```python
from build123d import *

# Parameters (mm, degrees)
SKETCH2_W                    = 28
SKETCH2_H                    = 8
BOSS_EXTRUDE1_DEPTH          = 2
SKETCH3_R                    = 2.35
BOSS_EXTRUDE2_DEPTH          = 10
CHAMFER1_SIZE                = 10
CHAMFER1_SIZE_2              = 0.3
LPATTERN1_COUNT              = 2
LPATTERN1_PITCH              = 20
CHAMFER1_OF_LPATTERN1_SIZE   = 10
CHAMFER1_OF_LPATTERN1_SIZE_2 = 0.3


with BuildPart() as part:
    # Sketch2 → Boss-Extrude1 (new body)
    with BuildSketch(Plane(origin=(0, 0, 0), x_dir=(1, 0, 0), z_dir=(0, 1, 0))):
        Rectangle(SKETCH2_W, SKETCH2_H)
    extrude(amount=BOSS_EXTRUDE1_DEPTH)

    # Sketch3 → Boss-Extrude2 (add)
    with BuildSketch(Plane(origin=(0, 2, 0), x_dir=(1, 0, 0), z_dir=(0, 1, 0))):
        with Locations(Location((10, 0, 0), (0, 0, 90))):
            Circle(SKETCH3_R)
    boss_extrude2 = extrude(amount=BOSS_EXTRUDE2_DEPTH)

    # Chamfer1
    # the kernel refuses this chamfer: 10, 0.3 mm, written as the material it takes off along each edge
    with BuildSketch(Plane(origin=(10, 12, 0), x_dir=(0, 0, -1), z_dir=(1, 0, 0))) as chamfer1_piece_1_section:
        Polygon((2.35, -CHAMFER1_SIZE), (2.35 - CHAMFER1_SIZE_2, 0), (2.35, 0), align=None)
    chamfer1_piece_1 = revolve(axis=Axis((10, 12, 0), (0, 1, 0)), mode=Mode.PRIVATE)
    chamfer1_piece_1 = split(chamfer1_piece_1, bisect_by=Plane(origin=(10, 2, 2.231636086), z_dir=(0, 1, 0)), keep=Keep.TOP, mode=Mode.PRIVATE)
    add(chamfer1_piece_1, mode=Mode.SUBTRACT)

    # LPattern1: Boss-Extrude2 ×2
    with Locations(*[(-i * LPATTERN1_PITCH, 0, 0) for i in range(1, LPATTERN1_COUNT)]):
        add(boss_extrude2)

    # Chamfer1 of LPattern1
    # the kernel refuses this chamfer: 10, 0.3 mm, written as the material it takes off along each edge
    with BuildSketch(Plane(origin=(-10, 12, 0), x_dir=(0, 0, -1), z_dir=(1, 0, 0))) as chamfer1_of_lpattern1_piece_1_section:
        Polygon((2.35, -CHAMFER1_OF_LPATTERN1_SIZE), (2.35 - CHAMFER1_OF_LPATTERN1_SIZE_2, 0), (2.35, 0), align=None)
    chamfer1_of_lpattern1_piece_1 = revolve(axis=Axis((-10, 12, 0), (0, 1, 0)), mode=Mode.PRIVATE)
    chamfer1_of_lpattern1_piece_1 = split(chamfer1_of_lpattern1_piece_1, bisect_by=Plane(origin=(-10, 2, 2.231636086), z_dir=(0, 1, 0)), keep=Keep.TOP, mode=Mode.PRIVATE)
    add(chamfer1_of_lpattern1_piece_1, mode=Mode.SUBTRACT)


solid = part.part
```
Input: part model. Units: mm. Frame: model coordinates. A direction names the side the tool comes from. Round coordinates to 2 decimals unless told otherwise and drop trailing zeros. Write each loop counter-clockwise with the first axis right and the second up, starting at its lowest first coordinate (ties: lowest second). Pieces come first, ordered by that corner, then holes. Notation, with made-up numbers: (89.5, 12) -> (115.5, 12) arc R18 cw to (115.5, 16) -> close; hole circle Ø2 at (35.25, 3). An arc over 180 degrees is marked (long way). Answer as CSV lines item,"result".
1. Reachability of faces 1 (the flat face through (-10, 12, 0)), 2 (the conical face through (-7.854, 7.07, 0.476)) from +Z, -Z, +X, -X, +Y, -Y: full face, straight path, thin tool, end or side. Return the list, or none.
Geometry says:
face 1,"+Z, -Z, +X, -X, +Y"
face 2,"+Y"
2. Contact query for flat-ended pins moving along their axis: P1, Ø1.5, axis at x = -6, z = -1.5, coming from the +Y side; P2, Ø3, axis at x = 5.5, z = 1, coming from the -Y side; P3, Ø3, axis at y = 4.5, z = -2.5, coming from the -X side. Output: stop coordinate, or through.
Geometry says:
P1,"stops at y = 2"
P2,"stops at y = 0"
P3,"stops at x = -12.05"
3. Section A-A (z = 0). Return the cut outline in (x, y), plus the area to 3 significant figures.
Geometry says:
outline,"(-14, 0) -> (14, 0) -> (14, 2) -> (12.35, 2) -> (12.05, 12) -> (7.95, 12) -> (7.65, 2) -> (-7.65, 2) -> (-7.95, 12) -> (-12.05, 12) -> (-12.35, 2) -> (-14, 2) -> close"
area,"144 mm^2"
4. Mould query, pull axis X, two halves, no side actions, for faces 3 (the flat face through (14, 1, 0)), 4 (the conical face through (12.146, 7.07, 0.476)), 5 (the flat face through (0, 0, 0)), 6 (the flat face through (-14, 1, 0)). Classes: +X half, -X half, draft (parallel to the pull), parting line (faces both ways), or undercut.
Geometry says:
face 3,"+X half"
face 4,"undercut"
face 5,"draft"
face 6,"-X half"
5. Ray query, L1, parallel to Y at x = 2, z = -2; L2, parallel to X at y = 5, z = -1.5; L3, parallel to X at y = 3, z = -0.25. Return the intervals inside material, ascending. Write a range as [from, to].
Geometry says:
L1,"y = [0, 2]"
L2,"x = [-11.69, -8.31], [8.31, 11.69]"
L3,"x = [-12.31, -7.69], [7.69, 12.31]"
6. Section C-C (x = -10). Return the cut outline in (y, z), plus the area to 3 significant figures.
Geometry says:
outline,"(0, -4) -> (2, -4) -> (2, -2.35) -> (12, -2.05) -> (12, 2.05) -> (2, 2.35) -> (2, 4) -> (0, 4) -> close"
area,"60.0 mm^2"
7. Section D-D (y = 10). Return the cut outline in (x, z).
Geometry says:
outline,"circle Ø4.22 at (-10, 0); circle Ø4.22 at (10, 0)"
8. Section B-B (y = 7). Return the cut outline in (x, z).
Geometry says:
outline,"circle Ø4.4 at (-10, 0); circle Ø4.4 at (10, 0)"
